```python
from build123d import *

# Parameters (mm, degrees)
SKETCH2_R            = 30
BOSS_EXTRUDE1_DEPTH  = 52.5
BOSS_EXTRUDE2_DEPTH  = 10
CUT_EXTRUDE1_DEPTH   = 430.890974551
SKETCH5_R            = 30
BOSS_EXTRUDE3_DEPTH  = 52.5
SKETCH6_R            = 50
BOSS_EXTRUDE4_DEPTH  = 10
FILLET1_R            = 10
FILLET1_OF_MIRROR3_R = 10


with BuildPart() as part:
    # Sketch2 → Boss-Extrude1 (new, symmetric)
    with BuildSketch(Plane.XY):
        Circle(SKETCH2_R)
    extrude(amount=BOSS_EXTRUDE1_DEPTH, both=True)

    # Sketch3 → Boss-Extrude2 (add)
    with BuildSketch(Plane.XY.offset(30)):
        with BuildLine():
            Line((0, 40), (380, 40))
            ThreePointArc((380, 40), (420, 0), (380, -40))
            Line((380, -40), (0, -40))
            ThreePointArc((0, -40), (-40, 0), (0, 40))
        make_face()
    boss_extrude2 = extrude(amount=-BOSS_EXTRUDE2_DEPTH)

    # Sketch4 → Cut-Extrude1 (cut, through all)
    with BuildSketch(Plane.XY.offset(30)):
        with BuildLine():
            Line((265, -25), (115, -25))
            ThreePointArc((115, -25), (90, 0), (115, 25))
            Line((115, 25), (265, 25))
            ThreePointArc((265, 25), (290, 0), (265, -25))
        make_face()
    cut_extrude1 = extrude(amount=-CUT_EXTRUDE1_DEPTH, mode=Mode.SUBTRACT)

    # Sketch5 → Boss-Extrude3 (add, symmetric)
    with BuildSketch(Plane.XY):
        with Locations((380, 0)):
            Circle(SKETCH5_R)
    extrude(amount=BOSS_EXTRUDE3_DEPTH, both=True)

    # Mirror1: Boss-Extrude2, Cut-Extrude1 across plane
    add(boss_extrude2.mirror(Plane.XY))
    add(cut_extrude1.mirror(Plane.XY), mode=Mode.SUBTRACT)

    # Sketch6 → Boss-Extrude4 (add)
    with BuildSketch(Plane.XY.offset(52.5)):
        Circle(SKETCH6_R)
        with Locations((380, 0)):
            Circle(SKETCH6_R)
    boss_extrude4 = extrude(amount=BOSS_EXTRUDE4_DEPTH)

    # Fillet1
    fillet1_edges = [part.edges().sort_by_distance(p)[0] for p in [
        (-50, 0, 62.5),
        (330, 0, 62.5),
    ]]
    fillet(fillet1_edges, radius=FILLET1_R - 0.0001)  # a hair under: the kernel refuses the full size

    # Mirror3: Boss-Extrude4 across plane
    add(boss_extrude4.mirror(Plane.XY))

    # Fillet1 of Mirror3
    fillet1_of_mirror3_edges = [part.edges().sort_by_distance(p)[0] for p in [
        (-50, 0, -62.5),
        (330, 0, -62.5),
    ]]
    fillet(fillet1_of_mirror3_edges, radius=FILLET1_OF_MIRROR3_R - 0.0001)  # a hair under: the kernel refuses the full size


solid = part.part
```
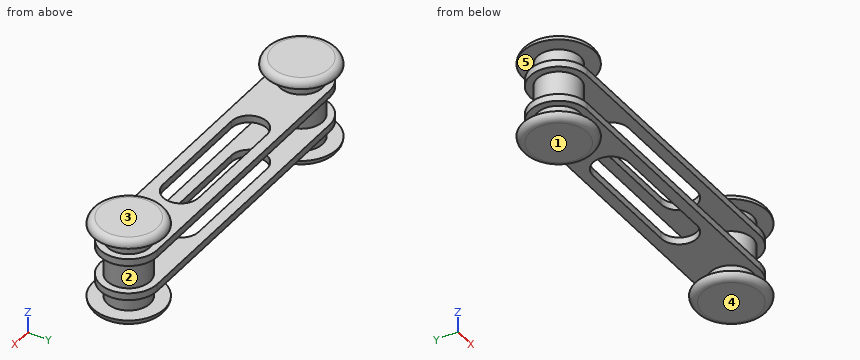
Model file for the job. Use its own axes, mm. Face numbers are marked on the shaded views. A direction names the side the tool comes from. Give positions to 0.01 mm unless a question says otherwise; leave off trailing zeros. Write each loop counter-clockwise with the first axis right and the second up, starting at its lowest first coordinate (ties: lowest second). Pieces come first, ordered by that corner, then holes. Notation, with made-up numbers: M 48.5,-16.5 L 99.5,-16.5 A22 cw 99.5,7.5 Z; hole C 40,4 d4. An arc over 180 degrees is marked long. Use a Markdown table: item, result.
1) Cut at A-A (x = 224). List the corners of the cut face in (y, z), and give its area (3 significant figures).
Responses:
| item | result |
|---|---|
| outline | M -40,-30 L -25,-30 L -25,-20 L -40,-20 Z; M -40,20 L -25,20 L -25,30 L -40,30 Z; M 25,-30 L 40,-30 L 40,-20 L 25,-20 Z; M 25,20 L 40,20 L 40,30 L 25,30 Z |
| area | 600 mm2 |
2) Tool access for the marked faces 4 and 5: list every direction of +Z, -Z, +X, -X, +Y, -Y with a clear straight run to the whole face (end or side of a thin tool).
Responses:
| item | result |
|---|---|
| face 4 | -Z, +X, -X, +Y, -Y |
| face 5 | none |
3) Drill centre lines: line 1 (Z direction, x = -25, y = -28); line 2 (Z direction, x = 330, y = -15.5); line 3 (X direction, y = -23.5, z = -7). Where is each one in solid material? Low to high. Write a range as from..to.
Responses:
| item | result |
|---|---|
| line 1 | z = -62.5..-52.5, -30..-20, 20..30, 52.5..62.5 |
| line 2 | z = -30..-20, 20..30 |
| line 3 | x = -18.65..18.65, 361.35..398.65 |
4) Pin check, flat tips, straight feed: pin 1 (1.5 mm diameter, centred on y = -3.5, z = -20.5, fed in from +X); pin 2 (10 mm diameter, centred on x = 56.5, y = 15.5, fed in from +Z); pin 3 (1 mm diameter, centred on x = 332.5, z = -22, fed in from -Y); pin 4 (24 mm diameter, centred on x = 241, y = -3, fed in from -Z). Stop position of each tip, or through.
Responses:
| item | result |
|---|---|
| pin 1 | stops at x = 419.91 |
| pin 2 | stops at z = 30 |
| pin 3 | stops at y = -40 |
| pin 4 | passes through |
5) Cut at B-B (z = -11.5). List the corners of the cut face in (x, y), and give its area (3 significant figures).
Responses:
| item | result |
|---|---|
| outline | C 0,0 d60; C 380,0 d60 |
| area | 5,650 mm2 |
6) Pull direction Z, two halves, no side cores. Call the marked faces 1, 2 and 3: +Z half, -Z half, draft (parallel to the pull), parting line (faces both ways), or undercut.
Responses:
| item | result |
|---|---|
| face 1 | -Z half |
| face 2 | undercut |
| face 3 | +Z half |
